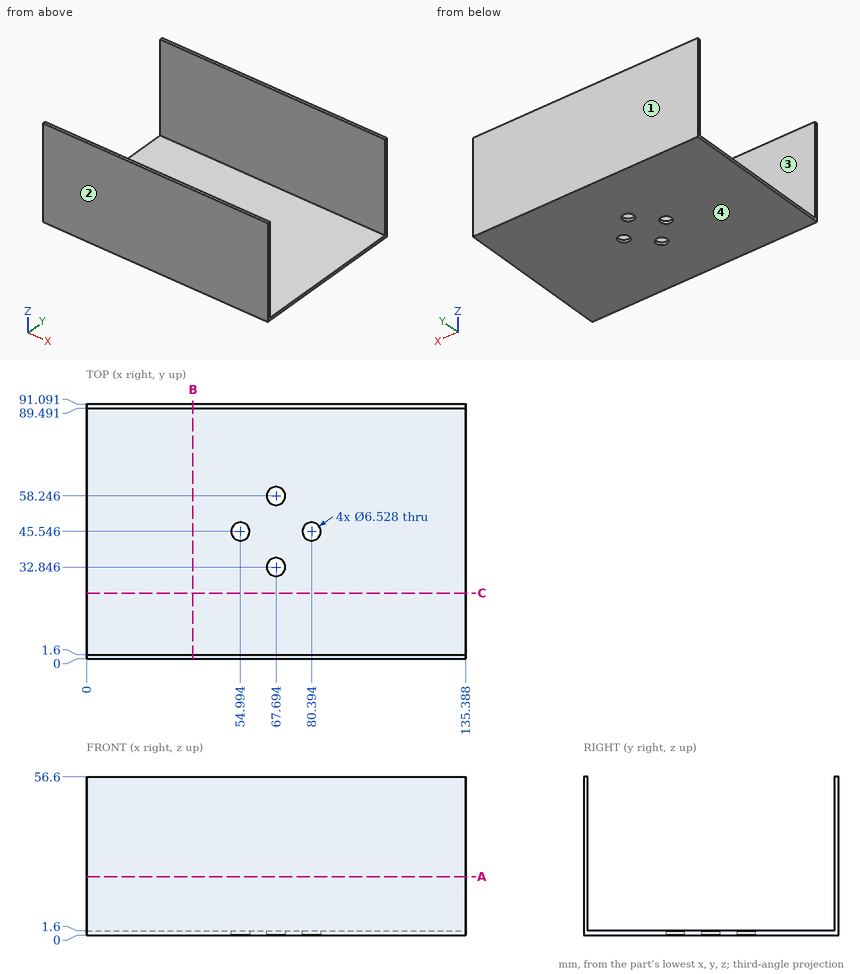
Can you work these out from the drawing? Everything is in mm from the part's minimum corner. Round coordinates to 2 decimals unless told otherwise and drop trailing zeros. Write each loop counter-clockwise with the first axis right and the second up, starting at its lowest first coordinate (ties: lowest second). Pieces come first, ordered by that corner, then holes.
1. If we mould it in two halves opening along Y, with no side actions, what happens to the marked faces 1, 2, 3 and 4? For each: released by +Y, released by -Y, zero draft, split by the parting line, or undercut.
2. Suppose I cut it at B-B (x = 38). List the corners of the cut face in (y, z) for me.
3. I need wall thicknesses on L1, parallel to Y at x = 53.5, z = 5.5; L2, parallel to Z at x = 50, y = 79. Which ranges of each line are inside material? Lowest first, please.
4. Suppose I cut it at A-A (z = 21). List the corners of the cut face in (x, y) for me.
5. Suppose I cut it at C-C (y = 23.5). List the corners of the cut face in (x, z) for me.
6. Will these pins go through, and if not, where does the flat tip stop? pin 1 Ø10.5 at (x, y) = (67.69, 58.25) entering from +Z; pin 2 Ø6 at (x, y) = (54.99, 45.55) entering from -Z.
Answer sheet:
1. face 1: released by +Y
1. face 2: released by -Y
1. face 3: undercut
1. face 4: zero draft
2. outline: (0, 0) - (91.09, 0) - (91.09, 56.6) - (89.49, 56.6) - (89.49, 1.6) - (1.6, 1.6) - (1.6, 56.6) - (0, 56.6) - close
3. L1: y = 0 to 1.6, 89.49 to 91.09
3. L2: z = 0 to 1.6
4. outline: (0, 0) - (135.39, 0) - (135.39, 1.6) - (0, 1.6) - close; (0, 89.49) - (135.39, 89.49) - (135.39, 91.09) - (0, 91.09) - close
5. outline: (0, 0) - (135.39, 0) - (135.39, 1.6) - (0, 1.6) - close
6. pin 1: stops at z = 1.6
6. pin 2: passes through
